```python
from build123d import *

# Parameters (mm, degrees)
F0_W      = 50
F0_H      = 17
F1_DEPTH  = 11
F2_W      = 37.7
F2_H      = 18.4
F3_DEPTH  = 12.5
F5_DEPTH  = 50.001
F6_W      = 6.15
F6_H      = 2.5
F7_DEPTH  = 10
F8_DEPTH  = 20
F9_W      = 6.15
F9_H      = 2
F10_DEPTH = 15.1
F11_W     = 9.5
F11_H     = 8
F12_DEPTH = 50.001
F13_W     = 6.15
F13_H     = 2
F14_DEPTH = 3
F15_SIZE  = 1.5


with BuildPart() as f1:
    # F0 (on Top) → F1 (new body)
    with BuildSketch(Plane.XY):
        Rectangle(F0_W, F0_H)
    extrude(amount=F1_DEPTH)

    # F2 (on Front) → F3 (cut, symmetric)
    with BuildSketch(Plane.XZ):
        Rectangle(F2_W, F2_H)
    extrude(amount=F3_DEPTH, both=True, mode=Mode.SUBTRACT)

    # F4 (on face) → F5 (cut, through all)
    with BuildSketch(Plane.YZ.offset(25)):
        with BuildLine():
            Line((1, 0), (1, 4))
            ThreePointArc((1, 4), (0, 5), (-1, 4))
            Line((-1, 4), (-1, 0))
            Line((-1, 0), (1, 0))
        make_face()
    extrude(amount=-F5_DEPTH, mode=Mode.SUBTRACT)

    # F6 (on face) → F7 (join)
    with BuildSketch(Plane.XY.offset(11)):
        with Locations((-21.925, -7.25)):
            Rectangle(F6_W, F6_H)
        with Locations((21.925, -7.25)):
            Rectangle(F6_W, F6_H)
    extrude(amount=F7_DEPTH)

    # F6 (on face) → F8 (join)
    with BuildSketch(Plane.XY.offset(11)):
        with Locations((-21.925, -7.25)):
            Rectangle(F6_W, F6_H)
        with Locations((21.925, -7.25)):
            Rectangle(F6_W, F6_H)
    extrude(amount=-F8_DEPTH)

    # F9 (on face) → F10 (join)
    with BuildSketch(Plane(origin=(0, -6, 0), x_dir=(-1, 0, 0), z_dir=(0, 1, 0))):
        with Locations((-21.925, -2.5)):
            Rectangle(F9_W, F9_H)
        with Locations((21.925, -2.5)):
            Rectangle(F9_W, F9_H)
    extrude(amount=F10_DEPTH)

    # F11 (on face) → F12 (cut, through all)
    with BuildSketch(Plane(origin=(-25, 0, 0), x_dir=(0, -1, 0), z_dir=(-1, 0, 0))):
        with Locations((-3.75, 4)):
            Rectangle(F11_W, F11_H)
    extrude(amount=-F12_DEPTH, mode=Mode.SUBTRACT)

    # F13 (on face) → F14 (join)
    with BuildSketch(Plane(origin=(0, 0, -3.5), x_dir=(1, 0, 0), z_dir=(0, 0, -1))):
        with Locations((21.925, -10.1)):
            Rectangle(F13_W, F13_H)
        with Locations((-21.925, -10.1)):
            Rectangle(F13_W, F13_H)
    extrude(amount=-F14_DEPTH)

    # F15
    f15_edges = [f1.edges().sort_by_distance(p)[0] for p in [
        (21.925, 11.1, -0.5),
        (-21.925, 11.1, -0.5),
    ]]
    chamfer(f15_edges, length=F15_SIZE)


solid = f1.part
```
Can you work these out from the model? Positions are in its coordinate system, mm. A direction names the side the tool comes from. Coordinates: 2 decimals unless noted, no trailing zeros. Loops run counter-clockwise (first coordinate to the right, second up) from the corner with the lowest first, then second, coordinate; pieces in that order, holes last. Notation, with made-up numbers: (12.25, 49.25) -> (35.25, 49.25) arc R24 ccw to (35.25, 73.25) -> close; hole circle Ø1 at (-13, 37.25). An arc over 180 degrees is marked (long way). Put each result on its own line as item: value. Start each with the question number.
Q1. I want a section at A-A (z = 12.5). Write out the boundary of the cut face in (x, y).
Q2. I'm going to push flat-ended pins straight in: P1, Ø3, axis at x = 14, y = 6, coming from the -Z side; P2, Ø1.6, axis at x = 21.5, z = -1, coming from the +Y side; P3, Ø8.5, axis at x = -11, y = 2, coming from the +Z side. Where does each tip first touch, or does it pass through?
Q3. I want a section at D-D (z = 3). Write out the boundary of the cut face in (x, y).
Q4. If I drill on line 1 (X direction, y = -7.25, z = 1); line 2 (Z direction, x = -21.5, y = 7); line 3 (Z direction, x = 12, y = 8), over which ranges is the centre line in solid material (lowest first)? Write a range as [from, to].
Q5. Thinking about a two-plate mould opening in X: for faces 1 (the face through (25, -3, 4)), 2 (the face through (-18.85, -7, 16)), 3 (the face through (-18.85, -3, 2)), 4 (the face through (-22, -7, 21)), which applies, pulls with the +X half, pulls with the -X half, needs draft (parallel to the pull), parting line crosses it, or undercut?
Q6. For faces 5 (the face through (-22, 10.4, -1.3)), 6 (the face through (22, 1, -1.5)), 7 (the face through (-22, 4, 8)), 8 (the face through (18.85, -7, 16)), 9 (the face through (-22, -6, -6)), which set-ups out of +Z, -Z, +X, -X, +Y, -Y let a thin tool reach every point of the face, with its end or its side?
Q7. I want a section at B-B (y = -1.5). Write out the boundary of the cut face in (x, z).
Q8. I want a section at C-C (x = -21). Write out the boundary of the cut face in (y, z).
Taken from the geometry:
1. outline: (-25, -8.5) -> (-18.85, -8.5) -> (-18.85, -6) -> (-25, -6) -> close; (18.85, -8.5) -> (25, -8.5) -> (25, -6) -> (18.85, -6) -> close
2. P1: stops at z = 9.2
2. P2: stops at y = 10.9
2. P3: stops at z = 11
3. outline: (-25, -8.5) -> (-18.85, -8.5) -> (-18.85, -1) -> (-25, -1) -> close; (18.85, -8.5) -> (25, -8.5) -> (25, -1) -> (18.85, -1) -> close
4. line 1: x = [-25, -18.85], [18.85, 25]
4. line 2: z = [-3.5, -1.5], [8, 11]
4. line 3: z = [9.2, 11]
5. face 1: pulls with the +X half
5. face 2: undercut
5. face 3: undercut
5. face 4: needs draft
6. face 5: +Z, +X, -X, +Y
6. face 6: +X, -X
6. face 7: +X, -X, +Y
6. face 8: +Z, +Y, -Y
6. face 9: -Z, +X, -X, +Y
7. outline: (-25, -3.5) -> (-18.85, -3.5) -> (-18.85, -1.5) -> (-25, -1.5) -> close; (-25, 0) -> (-18.85, 0) -> (-18.85, 9.2) -> (18.85, 9.2) -> (18.85, 0) -> (25, 0) -> (25, 11) -> (-25, 11) -> close; (18.85, -3.5) -> (25, -3.5) -> (25, -1.5) -> (18.85, -1.5) -> close
8. outline: (-8.5, -9) -> (-6, -9) -> (-6, -3.5) -> (11.1, -3.5) -> (11.1, -2) -> (9.6, -0.5) -> (9.1, -0.5) -> (9.1, -1.5) -> (-6, -1.5) -> (-6, 0) -> (-1, 0) -> (-1, 8) -> (8.5, 8) -> (8.5, 11) -> (-6, 11) -> (-6, 21) -> (-8.5, 21) -> close
